```python
from build123d import *

# Parameters (mm, degrees)
SKETCH1_W                = 34.714871787
SKETCH1_H                = 6
BOSS_EXTRUDE1_DEPTH      = 1
BOSS_EXTRUDE2_DEPTH      = 11
BOSS_EXTRUDE3_DEPTH      = 5
BOSS_EXTRUDE3_DEPTH_BACK = 3
SKETCH3_W                = 50
SKETCH3_H                = 7
CUT_EXTRUDE3_DEPTH       = 25
SKETCH5_W                = 50
SKETCH5_H                = 7
CUT_EXTRUDE4_DEPTH       = 25
SKETCH6_W                = 50
SKETCH6_H                = 7
CUT_EXTRUDE5_DEPTH       = 25
SKETCH8_R                = 1.500000001
SKETCH8_R_2              = 1.499999999
BOSS_EXTRUDE5_DEPTH      = 1
BOSS_EXTRUDE10_DEPTH     = 3


with BuildPart() as part:
    # Sketch1 → Boss-Extrude1 (new body)
    with BuildSketch(Plane(origin=(0, 0, 0), x_dir=(1, 0, 0), z_dir=(0, 1, 0))):
        Polygon((243.304219779, -116.484791863), (254.809280582, -136.408896135), (442.602090749, -136.409305398), (444.621046678, -132.925433226), (441.749040748, -132.925433226), (449.516726723, -119.47140646), (450.9646953, -121.978953126), (452.699916625, -118.984688022), (358.778179038, 43.666038061), (335.767496282, 43.666038061), align=None)
        with Locations((422.370878913, -131.984588005)):
            Rectangle(SKETCH1_W, SKETCH1_H, mode=Mode.SUBTRACT)
        Polygon((450.119365975, -117.364996826), (444.923425166, -120.365363323), (427.455346217, -90.114690822), (432.651287025, -87.114324326), align=None, mode=Mode.SUBTRACT)
        Polygon((428.11367092, -116.417164681), (266.439108269, -116.428009228), (347.27360973, 23.609230811), align=None, mode=Mode.SUBTRACT)
    extrude(amount=BOSS_EXTRUDE1_DEPTH)

    # Sketch1_9 → Boss-Extrude2 (add)
    # profile 1 of 2: a face of its own
    with BuildSketch(Plane(origin=(0, 0, 0), x_dir=(1, 0, 0), z_dir=(0, 1, 0))):
        Polygon((229.15943255, -134.984249185), (231.716666588, -139.412373829), (462.829865412, -139.412373829), (465.38624875, -134.984588004), (349.829542096, 65.165499075), (344.716133219, 65.165499075), align=None)
        Polygon((251.922647993, -136.409305396), (233.446303405, -136.408896135), (232.623553964, -134.984217354), (241.860901693, -118.984688015), align=None, mode=Mode.SUBTRACT)
        Polygon((442.602090749, -136.409305398), (254.809280582, -136.408896135), (243.304219779, -116.484791863), (335.767496282, 43.666038061), (358.778179038, 43.666038061), (461.93896796, -134.98458801), (461.116393748, -136.409305398), align=None, mode=Mode.SUBTRACT)
        Polygon((348.096628302, 62.164013367), (357.334800991, 46.166038067), (337.210874326, 46.166038067), (346.44844193, 62.165948237), align=None, mode=Mode.SUBTRACT)
    # profile 2 of 2: a face of its own
    with BuildSketch(Plane(origin=(0, 0, 0), x_dir=(1, 0, 0), z_dir=(0, 1, 0))):
        Polygon((441.749040748, -132.925433226), (444.621046678, -132.925433226), (450.9646953, -121.978953126), (449.516726723, -119.47140646), align=None)
    extrude(amount=BOSS_EXTRUDE2_DEPTH)

    # Sketch1_10 → Boss-Extrude3 (add, two sides: drawn at the far end of the back side and taken through both)
    # profile 1 of 2: a face of its own
    with BuildSketch(Plane(origin=(0, 0, 0), x_dir=(1, 0, 0), z_dir=(0, 1, 0)).offset(-BOSS_EXTRUDE3_DEPTH_BACK)):
        Polygon((229.15943255, -134.984249185), (231.716666588, -139.412373829), (462.829865412, -139.412373829), (465.38624875, -134.984588004), (349.829542096, 65.165499075), (344.716133219, 65.165499075), align=None)
        Polygon((251.922647993, -136.409305396), (233.446303405, -136.408896135), (232.623553964, -134.984217354), (241.860901693, -118.984688015), align=None, mode=Mode.SUBTRACT)
        Polygon((442.602090749, -136.409305398), (254.809280582, -136.408896135), (243.304219779, -116.484791863), (335.767496282, 43.666038061), (358.778179038, 43.666038061), (461.93896796, -134.98458801), (461.116393748, -136.409305398), align=None, mode=Mode.SUBTRACT)
        Polygon((348.096628302, 62.164013367), (357.334800991, 46.166038067), (337.210874326, 46.166038067), (346.44844193, 62.165948237), align=None, mode=Mode.SUBTRACT)
    # profile 2 of 2: a face of its own
    with BuildSketch(Plane(origin=(0, 0, 0), x_dir=(1, 0, 0), z_dir=(0, 1, 0)).offset(-BOSS_EXTRUDE3_DEPTH_BACK)):
        Polygon((441.749040748, -132.925433226), (444.621046678, -132.925433226), (450.9646953, -121.978953126), (449.516726723, -119.47140646), align=None)
    extrude(amount=BOSS_EXTRUDE3_DEPTH + BOSS_EXTRUDE3_DEPTH_BACK)

    # Sketch3 → Cut-Extrude3 (cut)
    with BuildSketch(Plane(origin=(290.589645397, 0, -167.772009994), x_dir=(-0.49999999999998745, 0, -0.8660254037844459), z_dir=(0.8660254037844459, 0, -0.49999999999998745))):
        with Locations((-236.592990632, -3)):
            Rectangle(SKETCH3_W, SKETCH3_H)
    extrude(amount=-CUT_EXTRUDE3_DEPTH, mode=Mode.SUBTRACT)

    # Sketch5 → Cut-Extrude4 (cut)
    with BuildSketch(Plane.XY.offset(139.412373829)):
        with Locations((347.273266, -3)):
            Rectangle(SKETCH5_W, SKETCH5_H)
    extrude(amount=-CUT_EXTRUDE4_DEPTH, mode=Mode.SUBTRACT)

    # Sketch6 → Cut-Extrude5 (cut)
    with BuildSketch(Plane(origin=(230.319375802, 0, 132.975171836), x_dir=(-0.5000006153901599, 0, 0.8660250484884727), z_dir=(-0.8660250484884727, 0, -0.5000006153901599))):
        with Locations((-113.236674797, -3)):
            Rectangle(SKETCH6_W, SKETCH6_H)
    extrude(amount=-CUT_EXTRUDE5_DEPTH, mode=Mode.SUBTRACT)

    # Sketch8 → Boss-Extrude5 (add)
    with BuildSketch(Plane.XZ.offset(3)):
        Polygon((349.829542096, -65.165499075), (465.38624875, 134.984588004), (462.829865412, 139.412373829), (231.716666588, 139.412373829), (229.15943255, 134.984249185), (344.716133219, -65.165499075), align=None)
        with Locations(Location((395.323540807, 98.692824233, 0), (0, 0, 270))):
            Circle(SKETCH8_R, mode=Mode.SUBTRACT)
        with Locations(Location((348.301285092, 15.86352663, 0), (0, 0, 270))):
            Circle(SKETCH8_R_2, mode=Mode.SUBTRACT)
        with Locations(Location((299.654911442, 97.241681778, 0), (0, 0, 270))):
            Circle(SKETCH8_R, mode=Mode.SUBTRACT)
        Polygon((444.621046678, 132.925433226), (450.9646953, 121.978953126), (449.516726723, 119.47140646), (427.347592194, 115.090208206), (404.332986149, 103.060878104), (405.774939108, 100.430142149), (424.549299543, 110.243170392), (451.871255231, 117.549638152), (452.699916625, 118.984688022), (461.93896796, 134.98458801), (461.116393748, 136.409305398), (442.602090749, 136.409305398), (439.019602541, 136.409297591), (420.379437569, 116.417683466), (402.410382204, 106.568526043), (403.852335163, 103.937790089), (426.620208945, 116.417264858), (441.749040748, 132.925433226), align=None, mode=Mode.SUBTRACT)
        Polygon((322.273266, 116.424264074), (294.35821863, 68.061097963), (319.354499369, 24.757680454), (376.473657314, 26.969372807), (401.472679509, 70.271207532), (372.273266, 116.420910254), align=None, mode=Mode.SUBTRACT)
        Polygon((233.446303405, 136.408896135), (251.922647993, 136.409305396), (241.860901693, 118.984688015), (232.623553964, 134.984217354), align=None, mode=Mode.SUBTRACT)
        Polygon((337.210874326, -46.166038067), (357.334800991, -46.166038067), (348.096628302, -62.164013367), (346.44844193, -62.165948237), align=None, mode=Mode.SUBTRACT)
    extrude(amount=BOSS_EXTRUDE5_DEPTH)

    # Sketch12 → Boss-Extrude10 (add)
    with BuildSketch(Plane(origin=(0, -3, 0), x_dir=(1, 0, 0), z_dir=(0, 1, 0))):
        with BuildLine():
            Line((347.417900212, -11.962292063), (347.307477102, -11.474637742))
            ThreePointArc((347.307477102, -11.474637741), (345.119304576, -12.681546115), (343.912396203, -14.86971864))
            Line((343.912396203, -14.86971864), (344.400050524, -14.98014175))
            ThreePointArc((344.400050524, -14.98014175), (345.472857967, -13.035099505), (347.417900212, -11.962292062))
        make_face()
        with BuildLine():
            ThreePointArc((352.690173981, -14.86971864), (351.483265607, -12.681546115), (349.295093082, -11.474637741))
            Line((349.295093082, -11.474637742), (349.184669972, -11.962292063))
            ThreePointArc((349.184669972, -11.962292062), (351.129712217, -13.035099505), (352.20251966, -14.98014175))
            Line((352.20251966, -14.98014175), (352.690173981, -14.86971864))
        make_face()
        with BuildLine():
            ThreePointArc((349.295093082, -20.25241552), (351.483265607, -19.045507146), (352.690173981, -16.85733462))
            Line((352.690173981, -16.85733462), (352.20251966, -16.74691151))
            ThreePointArc((352.20251966, -16.74691151), (351.129712217, -18.691953755), (349.184669972, -19.764761199))
            Line((349.184669972, -19.764761198), (349.295093082, -20.252415519))
        make_face()
        with BuildLine():
            Line((344.400050524, -16.74691151), (343.912396203, -16.85733462))
            ThreePointArc((343.912396203, -16.85733462), (345.119304576, -19.045507146), (347.307477102, -20.25241552))
            Line((347.307477102, -20.252415519), (347.417900212, -19.764761198))
            ThreePointArc((347.417900212, -19.764761199), (345.472857967, -18.691953755), (344.400050524, -16.74691151))
        make_face()
        with BuildLine():
            Line((394.440155927, -94.791589665), (394.329732817, -94.303935344))
            ThreePointArc((394.329732817, -94.303935343), (392.141560291, -95.510843717), (390.934651917, -97.699016243))
            Line((390.934651918, -97.699016243), (391.424789599, -97.798542944))
            ThreePointArc((391.424789599, -97.798542944), (392.499067688, -95.860448621), (394.440155927, -94.791589664))
        make_face()
        with BuildLine():
            ThreePointArc((399.712429696, -97.699016243), (398.505521322, -95.510843717), (396.317348797, -94.303935343))
            Line((396.317348797, -94.303935344), (396.206925687, -94.791589665))
            ThreePointArc((396.206925687, -94.791589664), (398.151967932, -95.864397108), (399.224775375, -97.809439353))
            Line((399.224775375, -97.809439353), (399.712429695, -97.699016243))
        make_face()
        with BuildLine():
            ThreePointArc((396.317348797, -103.081713122), (398.505521322, -101.874804748), (399.712429696, -99.686632223))
            Line((399.712429695, -99.686632223), (399.224775375, -99.576209113))
            ThreePointArc((399.224775375, -99.576209113), (398.151967932, -101.521251358), (396.206925687, -102.594058801))
            Line((396.206925687, -102.5940588), (396.317348797, -103.081713121))
        make_face()
        with BuildLine():
            Line((391.422306239, -99.576209113), (390.934651918, -99.686632223))
            ThreePointArc((390.934651917, -99.686632223), (392.141560291, -101.874804748), (394.329732817, -103.081713122))
            Line((394.329732817, -103.081713121), (394.440155927, -102.5940588))
            ThreePointArc((394.440155927, -102.594058801), (392.495113682, -101.521251358), (391.422306238, -99.576209113))
        make_face()
        with BuildLine():
            ThreePointArc((298.661103452, -92.85279289), (296.472930928, -94.059701263), (295.266022554, -96.247873788))
            Line((295.266022553, -96.247873788), (295.753676874, -96.358296898))
            ThreePointArc((295.753676875, -96.358296898), (296.826484318, -94.413254654), (298.771526562, -93.340447211))
            Line((298.771526562, -93.34044721), (298.661103452, -92.852792889))
        make_face()
        with BuildLine():
            ThreePointArc((304.04380033, -96.247873788), (302.836891957, -94.059701263), (300.648719432, -92.85279289))
            Line((300.648719432, -92.852792889), (300.538296322, -93.34044721))
            ThreePointArc((300.538296322, -93.340447211), (302.483338566, -94.413254654), (303.556146009, -96.358296898))
            Line((303.55614601, -96.358296898), (304.043800331, -96.247873788))
        make_face()
        with BuildLine():
            Line((300.538296322, -101.142916345), (300.648719432, -101.630570666))
            ThreePointArc((300.648719432, -101.630570665), (302.836891957, -100.423662292), (304.04380033, -98.235489767))
            Line((304.043800331, -98.235489768), (303.55614601, -98.125066658))
            ThreePointArc((303.556146009, -98.125066657), (302.483338566, -100.070108901), (300.538296322, -101.142916344))
        make_face()
        with BuildLine():
            Line((295.753676874, -98.125066658), (295.266022553, -98.235489768))
            ThreePointArc((295.266022554, -98.235489767), (296.472930928, -100.423662292), (298.661103452, -101.630570665))
            Line((298.661103452, -101.630570666), (298.771526562, -101.142916345))
            ThreePointArc((298.771526562, -101.142916344), (296.826484318, -100.070108901), (295.753676875, -98.125066657))
        make_face()
    extrude(amount=BOSS_EXTRUDE10_DEPTH)


solid = part.part
```
Model file for the job. Use its own axes, mm. A direction names the side the tool comes from. Round coordinates to 2 decimals unless told otherwise and drop trailing zeros. Order: outer loops, then holes, each group sorted by start corner. A loop starts at its lowest first (then second) coordinate and runs counter-clockwise, first axis right, second up. Notation, with made-up numbers: (-25.75, 5) -> (13.25, 5) arc R23 cw to (13.25, 25) -> close; hole circle Ø8 at (32, -9.75). An arc over 180 degrees is marked (long way). Use one line per item in the form item = value.
Item 1: Cut at A-A, the plane y = 3.75. Write the cut outline in (x, z), and give its area (3 significant figures).
Returned:
outline = (229.16, 134.98) -> (344.72, -65.17) -> (349.83, -65.17) -> (465.39, 134.98) -> (462.83, 139.41) -> (231.72, 139.41) -> close; (441.75, 132.93) -> (449.52, 119.47) -> (450.96, 121.98) -> (444.62, 132.93) -> close; hole (232.62, 134.98) -> (241.86, 118.98) -> (251.92, 136.41) -> (233.45, 136.41) -> close; hole (243.3, 116.48) -> (335.77, -43.67) -> (358.78, -43.67) -> (461.94, 134.98) -> (461.12, 136.41) -> (442.6, 136.41) -> (254.81, 136.41) -> close; hole (337.21, -46.17) -> (346.45, -62.17) -> (348.1, -62.16) -> (357.33, -46.17) -> close
area = 2,240 mm^2
Item 2: Cut at B-B, the plane x = 414. Give the number of separate pieces and of enclosed holes in the cut face, and give its area (3 significant figures).
Returned:
separate_pieces = 5
enclosed_holes = 0
area = 240 mm^2
Item 3: Pull direction X, two halves, no side cores. Call faces 5 (the face through (304.924, 0.168, 16.426)), 6 (the face through (434.08, -3.49, 124.56)), 7 (the face through (447, 11, 127)), 8 (the face through (259.934, -1.521, 87.681)): released by +X, released by -X, zero draft, split by the parting line, or undercut.
Returned:
face_5 = released by -X
face_6 = undercut
face_7 = zero draft
face_8 = undercut
Item 4: Flat gauge pins, fed straight in: pin 1 Ø1.1 at (y, z) = (0.5, 132) entering from +X; pin 2 Ø1.5 at (x, z) = (405, 71.5) entering from +Y; pin 3 Ø6 at (x, y) = (398, 6) entering from -Z. Where does each tip first touch, or does it go through?
Returned:
pin_1 = 463.98
pin_2 = 1
pin_3 = 13.07
Item 5: Drill centre lines: line 1 (Y direction, x = 277.5, z = 61.5); line 2 (Z direction, x = 431.5, y = -3.25); line 3 (Z direction, x = 353.5, y = 8.5). Where is each one in solid material? Low to high.
Returned:
line_1 = -4 to -3, 0 to 1
line_2 = 76.29 to 112.1, 115.91 to 121.74, 128.34 to 139.41
line_3 = -58.81 to -52.81, -46.17 to -43.67, 136.41 to 139.41
Item 6: Cut at C-C, the plane z = -49. Write the cut outline in (x, y), and give its area (3 significant figures).
Returned:
outline = (335.38, -4) -> (338.85, -4) -> (338.85, 11) -> (335.38, 11) -> close; (355.7, -4) -> (359.16, -4) -> (359.16, 11) -> (355.7, 11) -> close
area = 104 mm^2
Item 7: Tool access for faces 1 (the face through (341.894, 3.605, -54.278)), 2 (the face through (438.019, -3.493, 113.845)), 3 (the face through (445.69, -1.52, 126.1)), 4 (the face through (249.14, 5.93, 126.59)): list every direction of +Z, -Z, +X, -X, +Y, -Y with a clear straight run to the whole face (end or side of a thin tool).
Returned:
face_1 = +Y, -Y
face_2 = -Y
face_3 = none
face_4 = +Y
Item 8: Cut at D-D, the plane x = 312. Write the cut outline in (y, z).
Returned:
outline = (-4, -8.5) -> (11, -8.5) -> (11, -2.5) -> (1, -2.5) -> (1, 37.5) -> (0.5, 37.5) -> (0.5, 20.51) -> (0, 20.51) -> (0, -2.5) -> (-3, -2.5) -> (-3, 37.5) -> (-4, 37.5) -> close; (-4, 98.63) -> (-3, 98.63) -> (-3, 136.41) -> (0, 136.41) -> (0, 116.42) -> (1, 116.42) -> (1, 136.41) -> (11, 136.41) -> (11, 139.41) -> (-4, 139.41) -> close
